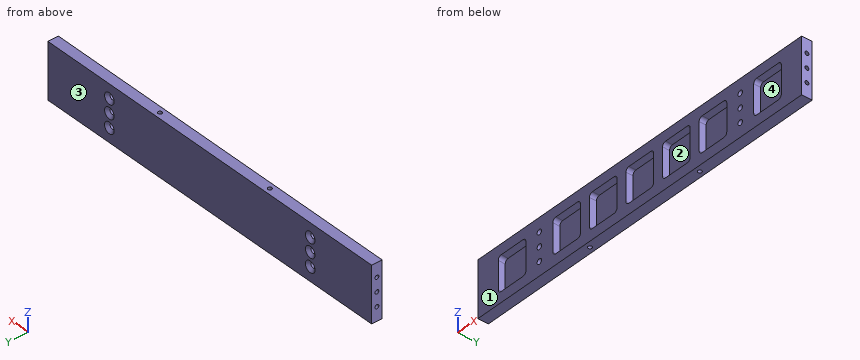
```python
from build123d import *

# Parameters (mm, degrees)
F0_W             = 342.9
F0_H             = 50.8
F1_DEPTH         = 9.525
F2_D             = 4.7625
F2_CSINK_D       = 10.16
F2_CSINK_ANGLE   = 90
F4_D             = 3.571875
F4_DEPTH         = 12.7
F4_TIP           = 1.0730995118
F6_D             = 3.571875
F6_DEPTH         = 12.7
F6_TIP           = 1.0730995118
F7_W             = 29.21
F7_H             = 31.75
F8_DEPTH         = 6.35
F9_R             = 3.175
F12_D            = 3.571875
F12_DEPTH        = 6.35
F12_TIP          = 1.0730995118
F12_ON_F10_D     = 3.571875
F12_ON_F10_DEPTH = 6.35
F12_ON_F10_TIP   = 1.0730995118


# Not quite as in the source:
# - a feature names something its author has since deleted; it is built from what else it names


with BuildPart() as f1:
    # F0 (on Front) → F1 (new body)
    with BuildSketch(Plane.XZ):
        with Locations((171.45, 25.4)):
            Rectangle(F0_W, F0_H)
    extrude(amount=F1_DEPTH)

    # F2 (through all)
    with Locations(Plane(origin=(0, 0, 0), x_dir=(1, 0, 0), z_dir=(0, 1, 0))):
        with Locations((65.0875, -38.1), (65.0875, -25.4), (65.0875, -12.7), (277.8125, -38.1), (277.8125, -25.4), (277.8125, -12.7)):
            CounterSinkHole(F2_D / 2, F2_CSINK_D / 2, counter_sink_angle=F2_CSINK_ANGLE)

    # F4
    with Locations(Plane(origin=(0, 0, 0), x_dir=(0, -1, 0), z_dir=(-1, 0, 0))):
        with Locations((4.7625, 25.4), (4.7625, 12.7), (4.7625, 38.1)):
            Hole(F4_D / 2, depth=F4_DEPTH)
            with Locations((0, 0, -(F4_DEPTH + F4_TIP / 2))):  # 118° drill point
                Cone(0, F4_D / 2, F4_TIP, mode=Mode.SUBTRACT)

    # F6
    with Locations(Plane.YZ.offset(342.9)):
        with Locations((-4.7625, 12.7), (-4.7625, 25.4), (-4.7625, 38.1)):
            Hole(F6_D / 2, depth=F6_DEPTH)
            with Locations((0, 0, -(F6_DEPTH + F6_TIP / 2))):  # 118° drill point
                Cone(0, F6_D / 2, F6_TIP, mode=Mode.SUBTRACT)

    # F7 (on face) → F8 (cut)
    with BuildSketch(Plane.XZ.offset(9.525)):
        with Locations((93.98, 25.4)):
            Rectangle(F7_W, F7_H)
        with Locations((132.715, 25.4)):
            Rectangle(F7_W, F7_H)
        with Locations((171.45, 25.4)):
            Rectangle(F7_W, F7_H)
        with Locations((210.185, 25.4)):
            Rectangle(F7_W, F7_H)
        with Locations((248.92, 25.4)):
            Rectangle(F7_W, F7_H)
        with Locations((36.195, 25.4)):
            Rectangle(F7_W, F7_H)
        with Locations((306.705, 25.4)):
            Rectangle(F7_W, F7_H)
    extrude(amount=-F8_DEPTH, mode=Mode.SUBTRACT)

    # F9
    f9_edges = [f1.edges().sort_by_distance(p)[0] for p in [
        (156.845, -6.35, 41.275),
        (195.58, -6.35, 41.275),
        (234.315, -6.35, 41.275),
        (79.375, -6.35, 41.275),
        (118.11, -6.35, 41.275),
        (79.375, -6.35, 9.525),
        (118.11, -6.35, 9.525),
        (156.845, -6.35, 9.525),
        (195.58, -6.35, 9.525),
        (234.315, -6.35, 9.525),
        (108.585, -6.35, 41.275),
        (147.32, -6.35, 41.275),
        (186.055, -6.35, 41.275),
        (224.79, -6.35, 41.275),
        (263.525, -6.35, 41.275),
        (263.525, -6.35, 9.525),
        (224.79, -6.35, 9.525),
        (186.055, -6.35, 9.525),
        (147.32, -6.35, 9.525),
        (108.585, -6.35, 9.525),
        (321.31, -6.35, 41.275),
        (292.1, -6.35, 41.275),
        (292.1, -6.35, 9.525),
        (321.31, -6.35, 9.525),
        (50.8, -6.35, 9.525),
        (50.8, -6.35, 41.275),
        (21.59, -6.35, 41.275),
        (21.59, -6.35, 9.525),
    ]]
    fillet(f9_edges, radius=F9_R)

    # F12
    with Locations(Plane.XY.offset(50.8)):
        with Locations((229.5525, -4.7625), (113.3475, -4.7625)):
            Hole(F12_D / 2, depth=F12_DEPTH)
            with Locations((0, 0, -(F12_DEPTH + F12_TIP / 2))):  # 118° drill point
                Cone(0, F12_D / 2, F12_TIP, mode=Mode.SUBTRACT)

    # F12 on F10
    with Locations(Plane(origin=(0, 0, 0), x_dir=(1, 0, 0), z_dir=(0, 0, -1))):
        with Locations((113.3475, 4.7625), (229.5525, 4.7625)):
            Hole(F12_ON_F10_D / 2, depth=F12_ON_F10_DEPTH)
            with Locations((0, 0, -(F12_ON_F10_DEPTH + F12_ON_F10_TIP / 2))):  # 118° drill point
                Cone(0, F12_ON_F10_D / 2, F12_ON_F10_TIP, mode=Mode.SUBTRACT)


solid = f1.part
```
Input: part model. Units: mm. Frame: model coordinates. Face numbers are marked on the shaded views. A direction names the side the tool comes from. Give positions to 0.01 mm unless a question says otherwise; leave off trailing zeros. Write each loop counter-clockwise with the first axis right and the second up, starting at its lowest first coordinate (ties: lowest second). Pieces come first, ordered by that corner, then holes. Notation, with made-up numbers: (76.25, 16.25) - (97.25, 16.25) arc R13 cw to (97.25, 25.25) - close; hole circle Ø9 at (38.5, 48). An arc over 180 degrees is marked (long way). Write item = value, one per line. Start each with the question number.
1) Pin query (flat end, axial travel): pin 1 (2 mm diameter, centred on y = -4.76, z = 25.4, fed in from +X); pin 2 (4.5 mm diameter, centred on x = 65.09, z = 25.4, fed in from +Y); pin 3 (6 mm diameter, centred on x = 277.81, z = 25.4, fed in from +Y); pin 4 (14.5 mm diameter, centred on x = 99.5, z = 25.5, fed in from -Y) (3 decimals). Return the tip coordinate at first contact, or that it passes through.
2) Material intervals for L1, parallel to Z at x = 127, y = -3.5 (3 decimals); L2, parallel to X at y = -2.5, z = 11.5; L3, parallel to Y at x = 94, z = 13 (3 decimals), sorted ascending. Write a range as [from, to].
3) Draft query along X for the marked faces 1 and 2. Return one class per face: pulls with the +X half, pulls with the -X half, needs draft (parallel to the pull), parting line crosses it, or undercut.
4) Cut plane A-A (x = 137). Return loops of the section in (y, z) (3 decimals), and give its area (3 significant figures).
5) Reachability of the marked faces 3 and 4 from +Z, -Z, +X, -X, +Y, -Y: full face, straight path, thin tool, end or side. Return the list, or none.
Answers follow:
q1.pin_1 = 329.73
q1.pin_2 = through
q1.pin_3 = -2.08
q1.pin_4 = -3.175
q2.L1 = [0, 9.525], [41.275, 50.8]
q2.L2 = [0, 62.8], [67.37, 275.53], [280.1, 342.9]
q2.L3 = [-3.175, 0]
q3.face_1 = needs draft
q3.face_2 = undercut
q4.outline = (-9.525, 0) - (0, 0) - (0, 50.8) - (-9.525, 50.8) - (-9.525, 41.275) - (-3.175, 41.275) - (-3.175, 9.525) - (-9.525, 9.525) - close
q4.area = 282 mm^2
q5.face_3 = +Z, -Z, +X, -X, +Y
q5.face_4 = -Y
